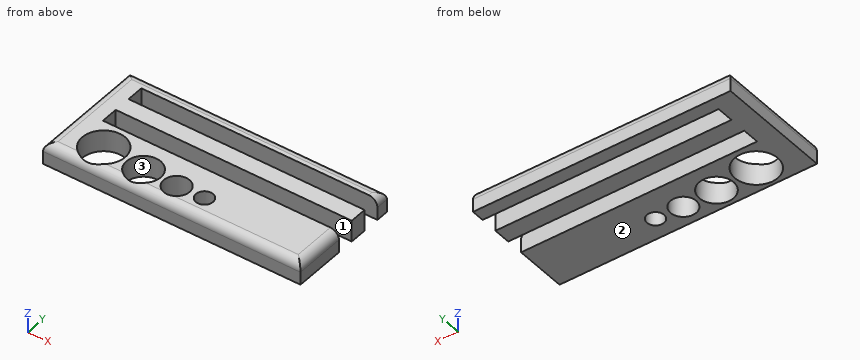
```python
from build123d import *

# Parameters (mm, degrees)
F0_R         = 6.35
F0_R_2       = 5.08
F0_R_3       = 3.81
F0_R_4       = 2.54
F1_DEPTH     = 6.35
F2_T1_DEPTH  = 88.9
F2_T3_DEPTH  = 46.99
F2_T5_DEPTH  = 10.16
F2_T10_DEPTH = 27.94


# Not quite as in the source:
# - a fillet or chamfer that OpenCascade refuses, or shapes differently, is made with other operations: its cross-section is extruded or revolved along the edge and cut away or added


with BuildPart() as f1:
    # F0 (on Top) → F1 (new body)
    with BuildSketch(Plane.XY):
        Polygon((-149.8234506369, 2.128423816), (-73.6234506369, 2.128423816), (-73.6234506369, 17.368423816), (-143.4734506369, 17.368423816), (-143.4734506369, 22.448423816), (-73.6234506369, 22.448423816), (-73.6234506369, 27.528423816), (-143.4734506369, 27.528423816), (-143.4734506369, 32.608423816), (-73.6234506369, 32.608423816), (-73.6234506369, 36.418423816), (-149.8234506369, 36.418423816), align=None)
        with Locations((-137.3288496289, 9.4627772336)):
            Circle(F0_R, mode=Mode.SUBTRACT)
        with Locations((-124.7644872946, 8.4292863984)):
            Circle(F0_R_2, mode=Mode.SUBTRACT)
        with Locations((-114.7297660142, 8.0924675546)):
            Circle(F0_R_3, mode=Mode.SUBTRACT)
        with Locations((-106.7409519207, 8.4292863984)):
            Circle(F0_R_4, mode=Mode.SUBTRACT)
    extrude(amount=F1_DEPTH)

    # F2: fillet of radius 2.54 on 5 edges, made by hand

    # F2_s2 → F2_t1 (cut)
    with BuildSketch(Plane.YZ.offset(-156.1734506369)):
        with BuildLine():
            ThreePointArc((36.418423816, 3.81), (35.6744750402, 5.6060512242), (33.878423816, 6.35))
            Line((33.878423816, 6.35), (36.418423816, 6.35))
            Line((36.418423816, 6.35), (36.418423816, 3.81))
        make_face()
        with BuildLine():
            ThreePointArc((2.128423816, 3.81), (2.8723725918, 5.6060512242), (4.668423816, 6.35))
            Line((4.668423816, 6.35), (2.128423816, 6.35))
            Line((2.128423816, 6.35), (2.128423816, 3.81))
        make_face()
    extrude(amount=F2_T1_DEPTH, mode=Mode.SUBTRACT)

    # F2_s4 → F2_t3 (cut)
    with BuildSketch(Plane.XZ.offset(-42.768423816)):
        with BuildLine():
            ThreePointArc((-149.8234506369, 3.81), (-149.0795018611, 5.6060512242), (-147.2834506369, 6.35))
            Line((-147.2834506369, 6.35), (-149.8234506369, 6.35))
            Line((-149.8234506369, 6.35), (-149.8234506369, 3.81))
        make_face()
    extrude(amount=F2_T3_DEPTH, mode=Mode.SUBTRACT)

    # F2_s6 → F2_t5 (cut)
    with BuildSketch(Plane.XZ.offset(-42.768423816)):
        with BuildLine():
            ThreePointArc((-73.6234506369, 3.81), (-74.3673994126, 5.6060512242), (-76.1634506369, 6.35))
            Line((-76.1634506369, 6.35), (-73.6234506369, 6.35))
            Line((-73.6234506369, 6.35), (-73.6234506369, 3.81))
        make_face()
    extrude(amount=F2_T5_DEPTH, mode=Mode.SUBTRACT)


with BuildPart() as f2_tool8:
    # F2_s9 → F2_t10 (new body)
    with BuildSketch(Plane.XZ.offset(4.221576184)):
        with BuildLine():
            ThreePointArc((-73.6234506369, 3.81), (-74.3673994126, 5.6060512242), (-76.1634506369, 6.35))
            Line((-76.1634506369, 6.35), (-73.6234506369, 6.35))
            Line((-73.6234506369, 6.35), (-73.6234506369, 3.81))
        make_face()
    extrude(amount=-F2_T10_DEPTH)

    split(bisect_by=Plane.XZ.offset(-22.448423816), keep=Keep.TOP)


with BuildPart() as f1_1:
    add(f1.part)

    # F2_t7: cut F2_tool8
    add(f2_tool8.part, mode=Mode.SUBTRACT)


solid = f1_1.part
```
Check sheet for the modelled part. Datum: model origin and axes. Units: mm. Face numbers are marked on the shaded views. Coordinates: 2 decimals unless noted, no trailing zeros. Write each loop counter-clockwise with the first axis right and the second up, starting at its lowest first coordinate (ties: lowest second). Pieces come first, ordered by that corner, then holes. Notation, with made-up numbers: (6, -29.75) -> (61, -29.75) arc R25 ccw to (61, 0.25) -> close; hole circle Ø4 at (-13.5, -19.75). An arc over 180 degrees is marked (long way). Use a Markdown table: item, result.
1. Sectioned sample at A-A (x = -90.5). Enter the section's corners in (y, z), plus the area to 3 significant figures.
Reported:
| item | result |
|---|---|
| outline | (2.13, 0) -> (17.37, 0) -> (17.37, 6.35) -> (4.67, 6.35) arc R2.54 ccw to (2.13, 3.81) -> close; (22.45, 0) -> (27.53, 0) -> (27.53, 6.35) -> (22.45, 6.35) -> close; (32.61, 0) -> (36.42, 0) -> (36.42, 3.81) arc R2.54 ccw to (33.88, 6.35) -> (32.61, 6.35) -> close |
| area | 150 mm2 |
2. Release check for a two-part mould opening along Y. For the marked faces 1, 2 and 3 record: pulls with the +Y half, pulls with the -Y half, needs draft (parallel to the pull), parting line crosses it, or undercut.
Reported:
| item | result |
|---|---|
| face 1 | undercut |
| face 2 | needs draft |
| face 3 | undercut |
3. Go/stop test with flat-tipped pins: pin 1 Ø3 at (x, z) = (-111.5, 4.5) entering from -Y; pin 2 Ø2.5 at (y, z) = (20.5, 2) entering from +X; pin 3 Ø8 at (x, y) = (-124.76, 8.43) entering from -Z; pin 4 Ø1 at (y, z) = (29.5, 4.5) entering from -X. Record where each tip stops, or that it passes through.
Reported:
| item | result |
|---|---|
| pin 1 | stops at y = 2.13 |
| pin 2 | stops at x = -143.47 |
| pin 3 | passes through |
| pin 4 | stops at x = -149.82 |
4. Sectioned sample at D-D (y = 29.5). Enter the section's corners in (x, z).
Reported:
| item | result |
|---|---|
| outline | (-149.82, 0) -> (-143.47, 0) -> (-143.47, 6.35) -> (-147.28, 6.35) arc R2.54 ccw to (-149.82, 3.81) -> close |
5. Sectioned sample at C-C (x = -114.5). Enter the section's corners in (y, z).
Reported:
| item | result |
|---|---|
| outline | (2.13, 0) -> (4.29, 0) -> (4.29, 6.32) arc R2.54 ccw to (2.13, 3.81) -> close; (11.9, 0) -> (17.37, 0) -> (17.37, 6.35) -> (11.9, 6.35) -> close; (22.45, 0) -> (27.53, 0) -> (27.53, 6.35) -> (22.45, 6.35) -> close; (32.61, 0) -> (36.42, 0) -> (36.42, 3.81) arc R2.54 ccw to (33.88, 6.35) -> (32.61, 6.35) -> close |
6. Scan lines: line 1 along Y through (x, z) = (-88.5, 1); line 2 along Y through (x, z) = (-106.5, 0.5); line 3 along Y through (x, z) = (-116, 2.75). Record each from-to range of solid material in increasing order.
Reported:
| item | result |
|---|---|
| line 1 | y = 2.13 to 17.37, 22.45 to 27.53, 32.61 to 36.42 |
| line 2 | y = 2.13 to 5.9, 10.96 to 17.37, 22.45 to 27.53, 32.61 to 36.42 |
| line 3 | y = 2.13 to 4.5, 11.68 to 17.37, 22.45 to 27.53, 32.61 to 36.42 |
7. Sectioned sample at B-B (z = 5.25). Enter the section's corners in (x, y), plus the area to 3 significant figures.
Reported:
| item | result |
|---|---|
| outline | (-149.38, 2.58) -> (-74.07, 2.58) -> (-74.07, 17.37) -> (-143.47, 17.37) -> (-143.47, 22.45) -> (-73.62, 22.45) -> (-73.62, 27.53) -> (-143.47, 27.53) -> (-143.47, 32.61) -> (-74.07, 32.61) -> (-74.07, 35.97) -> (-149.38, 35.97) -> close; hole circle Ø12.7 at (-137.33, 9.46); hole circle Ø10.16 at (-124.76, 8.43); hole circle Ø7.62 at (-114.73, 8.09); hole circle Ø5.08 at (-106.74, 8.43) |
| area | 1,540 mm2 |
